from build123d import *

# Parameters (mm, degrees)
SKETCH1_R           = 3.5
BOSS_EXTRUDE1_DEPTH = 7
SKETCH2_R           = 2.75
CUT_EXTRUDE1_DEPTH  = 7
FILLET2_R           = 0.3
FILLET3_R           = 0.3


with BuildPart() as part:
    # Sketch1 → Boss-Extrude1 (new body)
    with BuildSketch(Plane.XY):
        Circle(SKETCH1_R)
    extrude(amount=BOSS_EXTRUDE1_DEPTH)

    # Sketch2 → Cut-Extrude1 (cut)
    with BuildSketch(Plane(origin=(0, 0, 0), x_dir=(-1, 0, 0), z_dir=(0, 0, -1))):
        Circle(SKETCH2_R)
    extrude(amount=-CUT_EXTRUDE1_DEPTH, mode=Mode.SUBTRACT)

    # Fillet2
    fillet2_edges = [part.edges().sort_by_distance(p)[0] for p in [
        (-3.5, 0, 0),
        (2.75, 0, 7),
        (2.75, 0, 0),
    ]]
    fillet(fillet2_edges, radius=FILLET2_R)

    # Fillet3
    fillet3_edges = [part.edges().sort_by_distance(p)[0] for p in [
        (-3.5, 0, 7),
    ]]
    fillet(fillet3_edges, radius=FILLET3_R)


solid = part.part
Model file for the job. Use its own axes, mm. Coordinates: 2 decimals unless noted, no trailing zeros. Order: outer loops, then holes, each group sorted by start corner. A loop starts at its lowest first (then second) coordinate and runs counter-clockwise, first axis right, second up. Notation, with made-up numbers: M -39.5,-18.75 L -4.5,-18.75 A19 ccw -4.5,13.25 Z; hole C -24.75,3 d9. An arc over 180 degrees is marked long. Return JSON: item names as keys, results as strings.
1. Saw through at C-C (z = 5.25). Give the cut face in (x, y).
Ans:
{"outline": "C 0,0 d7; hole C 0,0 d5.5"}
2. Drill centre lines: probe 1 along Y at (x, z) = (0, 5.5); probe 2 along Y at (x, z) = (-1, 3.75); probe 3 along X at (y, z) = (1.5, 2.75). Where is each one in solid material? Low to high.
Ans:
{"probe 1": "-3.5 to -2.75, 2.75 to 3.5", "probe 2": "-3.35 to -2.56, 2.56 to 3.35", "probe 3": "-3.16 to -2.3, 2.3 to 3.16"}
3. Saw through at A-A (x = 0). Give the cut face in (y, z).
Ans:
{"outline": "M -3.5,0.3 A0.3 ccw -3.2,0 L -3.05,0 A0.3 ccw -2.75,0.3 L -2.75,6.7 A0.3 ccw -3.05,7 L -3.2,7 A0.3 ccw -3.5,6.7 Z; M 2.75,0.3 A0.3 ccw 3.05,0 L 3.2,0 A0.3 ccw 3.5,0.3 L 3.5,6.7 A0.3 ccw 3.2,7 L 3.05,7 A0.3 ccw 2.75,6.7 Z"}
4. Flat gauge pins, fed straight in: pin 1 (4 mm diameter, centred on y = -1.5, z = 3.5, fed in from -X); pin 2 (3 mm diameter, centred on x = 0.5, y = -1, fed in from +Z); pin 3 (3 mm diameter, centred on y = 2, z = 4, fed in from +X). Where does each tip first touch, or does it go through?
Ans:
{"pin 1": "x = -3.5", "pin 2": "through", "pin 3": "x = 3.46"}
